Source: CAD feature listing. Evaluate the final solid. Frame: model axes, mm. Face numbers are marked on the shaded views. A direction names the side the tool comes from. Coordinates: 2 decimals unless noted, no trailing zeros. Order: outer loops, then holes, each group sorted by start corner. A loop starts at its lowest first (then second) coordinate and runs counter-clockwise, first axis right, second up.
```python
from build123d import *

# Parameters (mm, degrees)
BOSS_EXTRUDE1_DEPTH = 3
BOSS_EXTRUDE2_DEPTH = 94
SKETCH4_R           = 1.4
SKETCH4_R_2         = 1.25
CUT_EXTRUDE1_DEPTH  = 2
SKETCH5_R           = 6.5
CUT_EXTRUDE2_DEPTH  = 2
SKETCH6_R           = 1
SKETCH6_R_2         = 1.25
CUT_EXTRUDE3_DEPTH  = 2
CUT_EXTRUDE4_DEPTH  = 2


with BuildPart() as part:
    # Sketch2 → Boss-Extrude1 (new body)
    with BuildSketch(Plane(origin=(0, 0, 0), x_dir=(1, 0, 0), z_dir=(0, 1, 0))):
        with BuildLine():
            Line((-43, 25.514701644), (-43, -25.514701644))
            ThreePointArc((-43, -25.514701644), (-37.211637523, -33.396018219), (-30, -40))
            Line((-30, -40), (-10, -40))
            Line((-10, -40), (-10, -48.989794856))
            ThreePointArc((-10, -48.989794856), (45.716299059, 20.248950598), (-43, 25.514701644))
        make_face()
    extrude(amount=BOSS_EXTRUDE1_DEPTH)

    # Sketch3 → Boss-Extrude2 (add)
    with BuildSketch(Plane(origin=(0, 3, 0), x_dir=(1, 0, 0), z_dir=(0, 1, 0))):
        with BuildLine():
            Line((-43, 25.514701644), (-43, -25.514701644))
            ThreePointArc((-43, -25.514701644), (-37.211637523, -33.396018219), (-30, -40))
            Line((-30, -40), (-10, -40))
            Line((-10, -40), (-10, -48.989794856))
            ThreePointArc((-10, -48.989794856), (45.716299059, 20.248950598), (-43, 25.514701644))
        make_face()
        with BuildLine():
            Line((-41, 24.959967949), (-41, -24.959967949))
            ThreePointArc((-41, -24.959967949), (-35.762251316, -32.01657978), (-29.325756597, -38))
            Line((-29.325756597, -38), (-10, -38))
            Line((-10, -38), (-10, 46.946778377))
            ThreePointArc((-10, 46.946778377), (-27.768776678, 39.152203537), (-41, 24.959967949))
        make_face(mode=Mode.SUBTRACT)
        with BuildLine():
            Line((-8, -38), (-8, -47.328638265))
            ThreePointArc((-8, -47.328638265), (-5.009902521, -47.737834856), (-2, -47.958315233))
            Line((-2, -47.958315233), (-2, 47.958315233))
            ThreePointArc((-2, 47.958315233), (-5.009902521, 47.737834856), (-8, 47.328638265))
            Line((-8, 47.328638265), (-8, -38))
        make_face(mode=Mode.SUBTRACT)
        with BuildLine():
            Line((0, 0), (0, 48))
            ThreePointArc((0, 48), (48, 0), (0, -48))
            Line((0, -48), (0, 0))
        make_face(mode=Mode.SUBTRACT)
    extrude(amount=BOSS_EXTRUDE2_DEPTH)

    # Sketch4 → Cut-Extrude1 (cut)
    with BuildSketch(Plane.ZY.offset(43)):
        with Locations((-9.75, 81.085264892)):
            Circle(SKETCH4_R)
        with Locations((9.75, 81.085264892)):
            Circle(SKETCH4_R)
        with Locations((0, 40.068908633)):
            Circle(SKETCH4_R_2)
        Polygon((0, 65.82), (10.87, 65.82), (10.87, 77), (-10.87, 77), (-10.87, 65.82), align=None)
        Polygon((-7.5, 55.590703336), (7.5, 55.590703336), (7.5, 51.590703336), (0, 51.590703336), (-7.5, 51.590703336), align=None)
        Polygon((0, 35.068908633), (6, 35.068908633), (6, 19.568908633), (-6, 19.568908633), (-6, 35.068908633), align=None)
    extrude(amount=-CUT_EXTRUDE1_DEPTH, mode=Mode.SUBTRACT)

    # Sketch5 → Cut-Extrude2 (cut)
    with BuildSketch(Plane.XY.offset(40)):
        with Locations((-19.974192729, 12)):
            Circle(SKETCH5_R)
    extrude(amount=-CUT_EXTRUDE2_DEPTH, mode=Mode.SUBTRACT)

    # Sketch6 → Cut-Extrude3 (cut)
    with BuildSketch(Plane.ZY.offset(10)):
        with Locations((-27.5, 82)):
            Circle(SKETCH6_R)
        with Locations((27.5, 82)):
            Circle(SKETCH6_R)
        with Locations((27.5, 9)):
            Circle(SKETCH6_R)
        with Locations((-27.5, 9)):
            Circle(SKETCH6_R)
        with Locations((-15, 88.839838551)):
            Circle(SKETCH6_R_2)
        with Locations((15, 88.839838551)):
            Circle(SKETCH6_R_2)
        with Locations((15, 58.839838551)):
            Circle(SKETCH6_R_2)
        with Locations((-15, 58.839838551)):
            Circle(SKETCH6_R_2)
        Polygon((-2.5, 95.222950519), (0, 95.222950519), (2.5, 95.222950519), (2.5, 90.222950519), (-2.5, 90.222950519), align=None)
    extrude(amount=-CUT_EXTRUDE3_DEPTH, mode=Mode.SUBTRACT)

    # Sketch7 → Cut-Extrude4 (cut)
    with BuildSketch(Plane.ZY.offset(2)):
        Polygon((-2.5, 93.960891169), (0, 93.960891169), (2.5, 93.960891169), (2.5, 88.960891169), (-2.5, 88.960891169), align=None)
    extrude(amount=-CUT_EXTRUDE4_DEPTH, mode=Mode.SUBTRACT)


solid = part.part
```
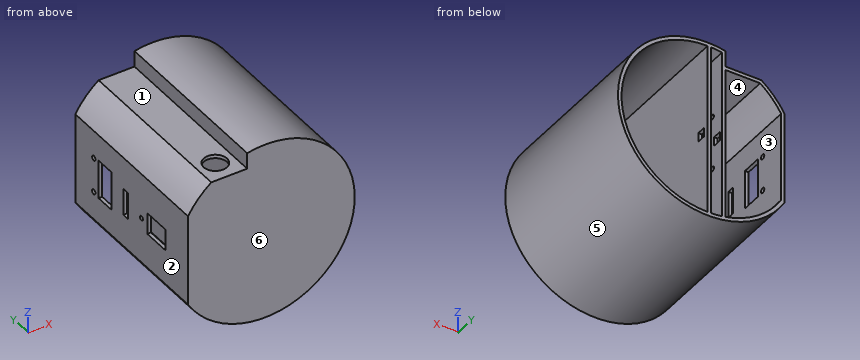
1. Draft query along Z for the marked faces 4, 5 and 6. Return one class per face: released by +Z, released by -Z, zero draft, split by the parting line, or undercut.
Findings:
face 4: undercut
face 5: split by the parting line
face 6: zero draft
2. Access query for the marked faces 1, 2 and 3. Directions: +Z, -Z, +X, -X, +Y, -Y. A direction counts if a zero-diameter tool reaches every point of the face in a straight line with its end or side. Return the directions, or none.
Findings:
face 1: +Z, -X, +Y, -Y
face 2: +Z, -Z, -X, +Y, -Y
face 3: +Y
3. Ray query, line 1 (Y direction, x = -9.3, z = -15); line 2 (Y direction, x = -41.75, z = 9.75); line 3 (X direction, y = 8, z = -6.5). Return the intervals inside material, ascending.
Findings:
line 1: y = 0 to 57.59, 60.09 to 87.59, 90.09 to 97
line 2: y = 0 to 65.82, 77 to 79.69, 82.49 to 97
line 3: x = -43 to -41, -10 to -8, -2 to 0, 47.56 to 49.58
4. Section query D-D on z = 19.5. Return loops of the section in (x, y).
Findings:
outline: (-43, 0) - (46.04, 0) - (46.04, 97) - (43.86, 97) - (43.86, 3) - (0, 3) - (0, 97) - (-2, 97) - (-2, 3) - (-8, 3) - (-8, 97) - (-10, 97) - (-10, 3) - (-41, 3) - (-41, 97) - (-43, 97) - close
5. Pin query (flat end, axial travel): P1, Ø5, axis at y = 13.5, z = 32, coming from the -X side; P2, Ø1.6, axis at x = -42, y = 29, coming from the -Z side; P3, Ø1, axis at x = -7, z = 9.5, coming from the +Y side. Return the tip coordinate at first contact, or that it passes through.
Findings:
P1: stops at x = -40.37
P2: stops at z = -28.33
P3: stops at y = 3
6. Section query A-A on y = 44. Return loops of the section in (x, z).
Findings:
outline: (-43, -25.51) arc R50 ccw (long way) to (-10, 48.99) - (-10, 40) - (-30, 40) arc R50 ccw to (-43, 25.51) - close; hole (-41, -24.96) arc R48 ccw to (-10, -46.95) - (-10, 38) - (-29.33, 38) arc R48 ccw to (-41, 24.96) - close; hole (-8, -47.33) arc R48 ccw to (-2, -47.96) - (-2, 47.96) arc R48 ccw to (-8, 47.33) - close; hole (0, -48) arc R48 ccw to (0, 48) - close
7. Section query B-B on y = 12. Return loops of the section in (x, z), plus the area to 3 significant figures.
Findings:
outline: (-43, -25.51) arc R50 ccw (long way) to (-10, 48.99) - (-10, 40) - (-13.47, 40) - (-13.47, 38) - (-10, 38) - (-10, -46.95) arc R48 cw to (-41, -24.96) - (-41, 24.96) arc R48 cw to (-29.33, 38) - (-26.47, 38) - (-26.47, 40) - (-30, 40) arc R50 ccw to (-43, 25.51) - close; hole (-8, -47.33) arc R48 ccw to (-2, -47.96) - (-2, 47.96) arc R48 ccw to (-8, 47.33) - close; hole (0, -48) arc R48 ccw to (0, 48) - close
area: 961 mm2
8. Section query C-C on x = -18. Return loops of the section in (y, z).
Findings:
outline: (0, -46.65) - (97, -46.65) - (97, -44.5) - (3, -44.5) - (3, 38) - (5.81, 38) - (5.81, 40) - (0, 40) - close; (18.19, 38) - (97, 38) - (97, 40) - (18.19, 40) - close
